```python
from build123d import *

# Parameters (mm, degrees)
SKETCH1_R                  = 2.2
SKETCH1_R_2                = 2.2479
EXTRUDE_BODY_DEPTH         = 4
SKETCH5_W                  = 10
SKETCH5_H                  = 10
SKETCH5_R                  = 2.2
SKETCH5_R_2                = 2.2479
EXTRUDE_LEGS_DEPTH         = 10
SKETCH6_R                  = 4.215
CUT_BOLT_HEAD_INSETS_DEPTH = 2.5


with BuildPart() as part:
    # Sketch1 → Extrude-Body (new body)
    with BuildSketch(Plane(origin=(0, 0, 0), x_dir=(1, 0, 0), z_dir=(0, 1, 0))):
        with BuildLine():
            Line((10, -10), (10, 10))
            Line((10, 10), (55, 10))
            Line((55, 10), (55, 32))
            Line((55, 32), (45, 32))
            ThreePointArc((45, 32), (27.5, 21), (10, 32))
            Line((10, 32), (0, 32))
            Line((0, 32), (0, -32))
            Line((0, -32), (10, -32))
            ThreePointArc((10, -32), (27.5, -21), (45, -32))
            Line((45, -32), (55, -32))
            Line((55, -32), (55, -10))
            Line((55, -10), (10, -10))
        make_face()
        with Locations(Location((50, 27, 0), (0, 0, 270))):
            Circle(SKETCH1_R, mode=Mode.SUBTRACT)
        with Locations(Location((50, -27, 0), (0, 0, 270))):
            Circle(SKETCH1_R, mode=Mode.SUBTRACT)
        with Locations(Location((5, 26.25, 0), (0, 0, 270))):
            Circle(SKETCH1_R_2, mode=Mode.SUBTRACT)
        with Locations(Location((5, -26.25, 0), (0, 0, 270))):
            Circle(SKETCH1_R_2, mode=Mode.SUBTRACT)
    extrude(amount=EXTRUDE_BODY_DEPTH)

    # Sketch5 → Extrude-Legs (add)
    # profile 1 of 4: a face of its own
    with BuildSketch(Plane(origin=(0, 4, 0), x_dir=(1, 0, 0), z_dir=(0, 1, 0))):
        with Locations((50, -27)):
            Rectangle(SKETCH5_W, SKETCH5_H)
        with Locations(Location((50, -27, 0), (0, 0, 270))):
            Circle(SKETCH5_R, mode=Mode.SUBTRACT)
    # profile 2 of 4: a face of its own
    with BuildSketch(Plane(origin=(0, 4, 0), x_dir=(1, 0, 0), z_dir=(0, 1, 0))):
        with Locations((50, 27)):
            Rectangle(SKETCH5_W, SKETCH5_H)
        with Locations(Location((50, 27, 0), (0, 0, 270))):
            Circle(SKETCH5_R, mode=Mode.SUBTRACT)
    # profile 3 of 4: a face of its own
    with BuildSketch(Plane(origin=(0, 4, 0), x_dir=(1, 0, 0), z_dir=(0, 1, 0))):
        with Locations((5, 27)):
            Rectangle(SKETCH5_W, SKETCH5_H)
        with Locations(Location((5, 26.25, 0), (0, 0, 270))):
            Circle(SKETCH5_R_2, mode=Mode.SUBTRACT)
    # profile 4 of 4: a face of its own
    with BuildSketch(Plane(origin=(0, 4, 0), x_dir=(1, 0, 0), z_dir=(0, 1, 0))):
        with Locations((5, -27)):
            Rectangle(SKETCH5_W, SKETCH5_H)
        with Locations(Location((5, -26.25, 0), (0, 0, 270))):
            Circle(SKETCH5_R_2, mode=Mode.SUBTRACT)
    extrude(amount=EXTRUDE_LEGS_DEPTH)

    # Sketch6 → Cut-Bolt Head Insets (cut)
    with BuildSketch(Plane.XZ):
        with Locations(Location((50, 27, 0), (0, 0, 270))):
            Circle(SKETCH6_R)
        with Locations(Location((50, -27, 0), (0, 0, 270))):
            Circle(SKETCH6_R)
    extrude(amount=-CUT_BOLT_HEAD_INSETS_DEPTH, mode=Mode.SUBTRACT)


solid = part.part
```
Here's how the part is built. I have some questions about the finished solid (model axes, mm). A direction names the side the tool comes from. Coordinates: 2 decimals unless noted, no trailing zeros. Loops run counter-clockwise (first coordinate to the right, second up) from the corner with the lowest first, then second, coordinate; pieces in that order, holes last. Notation, with made-up numbers: (85, 75.25) - (93, 75.25) arc R21 ccw to (93, 103.25) - close; hole circle Ø10 at (-34.75, 16). An arc over 180 degrees is marked (long way). Answer as CSV lines item,"result".
Q1. For pin 1 (13.5 mm diameter, centred on x = 50, z = -27, fed in from +Y); pin 2 (6 mm diameter, centred on x = 29, z = -17, fed in from +Y); pin 3 (2 mm diameter, centred on y = 1, z = 0, fed in from +X); pin 4 (1 mm diameter, centred on x = 16, y = 3.5, fed in from -Z), each with a flat end and sliding along its axis, tell me the tip position at first contact or that it passes through.
Response:
pin 1,"y = 14"
pin 2,"y = 4"
pin 3,"x = 10"
pin 4,"z = -25.15"
Q2. If we section it at A-A, the plane y = 5.5: Write out the boundary of the cut face in (x, z).
Response:
outline,"(0, -32) - (10, -32) - (10, -22) - (0, -22) - close; (0, 22) - (10, 22) - (10, 32) - (0, 32) - close; (45, -32) - (55, -32) - (55, -22) - (45, -22) - close; (45, 22) - (55, 22) - (55, 32) - (45, 32) - close; hole circle Ø4.5 at (5, -26.25); hole circle Ø4.5 at (5, 26.25); hole circle Ø4.4 at (50, -27); hole circle Ø4.4 at (50, 27)"
Q3. If we section it at C-C, the plane x = 21: Write out the boundary of the cut face in (y, z).
Response:
outline,"(0, -22.12) - (4, -22.12) - (4, -10) - (0, -10) - close; (0, 10) - (4, 10) - (4, 22.12) - (0, 22.12) - close"
Q4. We'd pull the mould along Z, two halves only. Please class faces 6 (the face through (33, 2, 10)), 7 (the face through (27.805, 1.972, -21.002)), 8 (the face through (55, 5, -23)), 9 (the face through (27.195, 1.972, 21.002)): pulls with the +Z half, pulls with the -Z half, needs draft (parallel to the pull), parting line crosses it, or undercut.
Response:
face 6,"undercut"
face 7,"pulls with the -Z half"
face 8,"needs draft"
face 9,"pulls with the +Z half"
Q5. For faces 1 (the face through (5.099, 6.902, 24.004)), 2 (the face through (5, 9, 22)), 3 (the face through (10, 9, -27)), 4 (the face through (50, 7, 32)), 5 (the face through (48, 2.5, 25)), which set-ups out of +Z, -Z, +X, -X, +Y, -Y let a thin tool reach every point of the face, with its end or its side?
Response:
face 1,"+Y, -Y"
face 2,"+X, -X, +Y"
face 3,"+Z, -Z, +Y"
face 4,"+Z, +X, -X, +Y, -Y"
face 5,"-Y"
Q6. If we section it at D-D, the plane z = 13: Write out the boundary of the cut face in (x, y).
Response:
outline,"(0, 0) - (55, 0) - (55, 4) - (0, 4) - close"
Q7. If I drill on L1, parallel to Z at x = 50, y = 11.5; L2, parallel to Z at x = 47, y = 13; L3, parallel to Z at x = 3.5, y = 9, over which ranges is the centre line in solid material (lowest first)? Write a range as [from, to].
Response:
L1,"[-32, -29.2], [-24.8, -22], [22, 24.8], [29.2, 32]"
L2,"[-32, -22], [22, 32]"
L3,"[-32, -27.92], [-24.58, -22], [22, 24.58], [27.92, 32]"
Q8. If we section it at B-B, the plane z = 27: Write out the boundary of the cut face in (x, y) (3 decimals), and give its area (3 significant figures).
Response:
outline,"(0, 0) - (2.881, 0) - (2.881, 14) - (0, 14) - close; (7.119, 0) - (13.463, 0) - (13.463, 4) - (10, 4) - (10, 14) - (7.119, 14) - close; (41.537, 0) - (45.785, 0) - (45.785, 2.5) - (47.8, 2.5) - (47.8, 14) - (45, 14) - (45, 4) - (41.537, 4) - close; (52.2, 2.5) - (54.215, 2.5) - (54.215, 0) - (55, 0) - (55, 14) - (52.2, 14) - close"
area,"177 mm2"
